from build123d import *

# Parameters (mm, degrees)
CHAMFER1_SIZE      = 2
CUT_EXTRUDE1_DEPTH = 5


with BuildPart() as part:
    # Sketch1 → Revolve1 (revolve)
    with BuildSketch(Plane.XY):
        Polygon((0, 0), (0, 22.5), (65, 22.5), (65, 27), (70, 27), (70, 52), (80, 52), (80, 35), (145, 35), (145, 52), (155, 52), (155, 24.5), (164, 24.5), (164, 21), (224, 21), (224, 0), align=None)
    revolve(axis=Axis((0, 0, 0), (1, 0, 0)))

    # Chamfer1
    chamfer1_edges = [part.edges().sort_by_distance(p)[0] for p in [
        (155, -24.5, 0),
        (145, -35, 0),
        (80, -35, 0),
    ]]
    chamfer(chamfer1_edges, length=CHAMFER1_SIZE)

    # Sketch2 → Cut-Extrude1 (cut)
    with BuildSketch(Plane(origin=(0, 21, 0), x_dir=(1, 0, 0), z_dir=(0, 1, 0))):
        with BuildLine():
            Line((194, 6), (194, -6))
            Line((194, -6), (174, -6))
            ThreePointArc((174, -6), (168, 0), (174, 6))
            Line((174, 6), (194, 6))
        make_face()
    cut_extrude1 = extrude(amount=-CUT_EXTRUDE1_DEPTH, mode=Mode.SUBTRACT)

    # Mirror1: Cut-Extrude1 across plane
    add(cut_extrude1.mirror(Plane(origin=(194, 16, -6), x_dir=(0, 0, 1), z_dir=(1, 0, 0))), mode=Mode.SUBTRACT)


solid = part.part
Geometry check sheet. Reference: the model listing, model coordinates, mm. A direction names the side the tool comes from. Coordinates: 2 decimals unless noted, no trailing zeros. Loops run counter-clockwise (first coordinate to the right, second up) from the corner with the lowest first, then second, coordinate; pieces in that order, holes last. Notation, with made-up numbers: (22.5, 69.5) - (26.5, 69.5) arc R24 cw to (26.5, 90.5) - close; hole circle Ø9 at (87.25, -5). An arc over 180 degrees is marked (long way). Use one line per item in the form item = value. Start each with the question number.
Item 1: Section check C-C, the plane x = 137. Enter the section's corners in (y, z).
Item 2: Thickness scan on probe 1 along X at (y, z) = (43.5, -16); probe 2 along X at (y, z) = (11, -21); probe 3 along X at (y, z) = (29, 11.5). Record the ranges inside material, lowest first.
Item 3: Gauge pin test, flat ends, axial feed: pin 1 (4 mm diameter, centred on x = 95, y = -7.5, fed in from +Z); pin 2 (3.5 mm diameter, centred on x = 204, z = -3, fed in from +Y); pin 3 (4.5 mm diameter, centred on x = 195, y = 17.5, fed in from +Z). Record the tip position at first contact, or that the pin passes through.
Item 4: Mould release check, pull along Z, two halves, no side actions. Record for faces 4 (the face through (164, 20, 7)), 5 (the face through (143.125, 33.503, 10.551)), 6 (the face through (220, 19, 0)): +Z half, -Z half, draft (parallel to the pull), parting line (faces both ways), or undercut.
Item 5: Section check B-B, the plane z = 42.5. Enter the section's corners in (x, y), and give its area (3 significant figures).
Item 6: Tool access check on faces 1 (the face through (194, 18, -6)), 2 (the face through (80, -12.3, 35.4)), 3 (the face through (160.55, 13.17, 20.66)). Record the directions out of +Z, -Z, +X, -X, +Y, -Y that give a thin tool (end or side, any length) a straight path to the whole face; none if there is none.
Computed:
q1.outline = circle Ø70 at (0, 0)
q2.probe_1 = 70 to 80, 145 to 155
q2.probe_2 = 65 to 164
q2.probe_3 = 70 to 155
q3.pin_1 = 34.57
q3.pin_2 = 16
q3.pin_3 = 14.44
q4.face_4 = draft
q4.face_5 = parting line
q4.face_6 = undercut
q5.outline = (70, -29.96) - (80, -29.96) - (80, 29.96) - (70, 29.96) - close; (145, -29.96) - (155, -29.96) - (155, 29.96) - (145, 29.96) - close
q5.area = 1,200 mm2
q6.face_1 = +Y
q6.face_2 = none
q6.face_3 = +X
